Check sheet for the modelled part. Datum: model origin and axes. Units: mm. Give positions to 0.01 mm unless a question says otherwise; leave off trailing zeros. Order: outer loops, then holes, each group sorted by start corner. A loop starts at its lowest first (then second) coordinate and runs counter-clockwise, first axis right, second up.
```python
from build123d import *

# Parameters (mm, degrees)
EXTRUDE_1_DEPTH     = 6
SKETCH_2_R          = 7
CUT_EXTRUDE_1_DEPTH = 103.099676082
FILLET_2_R          = 40
FILLET_3_R          = 10


with BuildPart() as part:
    # Эскиз1 → Бобышка-Вытянуть1 (new body)
    with BuildSketch(Plane.XY):
        Polygon((0, 0), (0, 80), (50, 88.816349035), (50, 0), align=None)
    extrude(amount=EXTRUDE_1_DEPTH)

    # Эскиз2 → Вырез-Вытянуть1 (cut, through all)
    with BuildSketch(Plane.XY):
        with Locations((19, 58.1)):
            Circle(SKETCH_2_R)
        with Locations((19, 20)):
            Circle(SKETCH_2_R)
    extrude(amount=CUT_EXTRUDE_1_DEPTH, mode=Mode.SUBTRACT)

    # Скругление2
    fillet_2_edges = [part.edges().sort_by_distance(p)[0] for p in [
        (50, 0, 3),
    ]]
    fillet(fillet_2_edges, radius=FILLET_2_R)

    # Скругление3
    fillet_3_edges = [part.edges().sort_by_distance(p)[0] for p in [
        (0, 0, 3),
    ]]
    fillet(fillet_3_edges, radius=FILLET_3_R - 0.0001)  # a hair under: the kernel refuses the full size


solid = part.part
```
(1) Release check for a two-part mould opening along Y. For faces 1 (the face through (50, 65, 3)), 2 (the face through (13.445, 15.741, 2.958)), 3 (the face through (37.972, 11.406, 3.042)) record: released by +Y, released by -Y, zero draft, split by the parting line, or undercut.
(2) Go/stop test with flat-tipped pins: P1, Ø3, axis at x = 40.5, z = 4, coming from the +Y side; P2, Ø3, axis at x = 20, z = 5, coming from the -Y side. Record where each tip stops, or that it passes through.
(3) Sectioned sample at C-C (x = 19). Enter the section's corners in (y, z), plus the area to 3 significant figures.
(4) Sectioned sample at D-D (y = 20). Enter the section's corners in (x, z), plus the area to 3 significant figures.
(5) Sectioned sample at B-B (z = 4.1). Count the separate pieces of the cut face and the enclosed holes in it, plus the area to 3 significant figures.
(6) Sectioned sample at A-A (y = 58.1). Enter the section's corners in (x, z).
(7) Thickness scan on L1, parallel to Y at x = 14, z = 1.7; L2, parallel to Y at x = 18, z = 1.4; L3, parallel to X at y = 20, z = 2.4. Record the ranges inside material, lowest first.
Values follow:
1. face 1: zero draft
1. face 2: undercut
1. face 3: released by -Y
2. P1: stops at y = 87.41
2. P2: stops at y = 0.91
3. outline: (1.03, 0) - (13, 0) - (13, 6) - (1.03, 6) - close; (27, 0) - (51.1, 0) - (51.1, 6) - (27, 6) - close; (65.1, 0) - (83.35, 0) - (83.35, 6) - (65.1, 6) - close
3. area: 326 mm2
4. outline: (0, 0) - (12, 0) - (12, 6) - (0, 6) - close; (26, 0) - (44.64, 0) - (44.64, 6) - (26, 6) - close
4. area: 184 mm2
5. separate pieces: 1
5. enclosed holes: 2
5. area: 3,550 mm2
6. outline: (0, 0) - (12, 0) - (12, 6) - (0, 6) - close; (26, 0) - (50, 0) - (50, 6) - (26, 6) - close
7. L1: y = 0.2 to 15.1, 24.9 to 53.2, 63 to 82.47
7. L2: y = 0.81 to 13.07, 26.93 to 51.17, 65.03 to 83.17
7. L3: x = 0 to 12, 26 to 44.64
